The listing builds one solid part. Answer for the finished solid, in the listing's coordinates (mm). A direction names the side the tool comes from. Coordinates: 2 decimals unless noted, no trailing zeros. Write each loop counter-clockwise with the first axis right and the second up, starting at its lowest first coordinate (ties: lowest second). Pieces come first, ordered by that corner, then holes. Notation, with made-up numbers: M 40,23.5 L 69,23.5 A21 ccw 69,27.5 Z; hole C 21,86.5 d10. An arc over 180 degrees is marked long. Answer as CSV lines item,"result". Start each with the question number.
```python
from build123d import *
from build123d.topology import SkipClean

# Parameters (mm, degrees)
CUT_EXTRUDE1_START = -254
CUT_EXTRUDE1_DEPTH = 254
CHAMFER1_SIZE      = 10
CHAMFER2_SIZE      = 10
CHAMFER3_SIZE      = 10
CHAMFER4_SIZE      = 10
FILLET1_R          = 10


with BuildPart() as part:
    # Sketch1 → Revolve4 (revolve)
    with BuildSketch(Plane.XY):
        Polygon((-381, 4.199357945), (-381, 80.399357945), (0, 80.399357945), (0, 105.799357945), (127, 105.799357945), (127, 118.499357945), (431.8, 118.499357945), (431.8, 105.799357945), (482.6, 105.799357945), (482.6, 80.399357945), (685.8, 80.399357945), (685.8, 4.199357945), align=None)
    revolve(axis=Axis((685.8, 4.199357945, 0), (-1, 0, 0)))

    # Sketch3 → Cut-Extrude1 (cut)
    with SkipClean():  # the faces are left unmerged after this step: merging them gives an invalid solid
        with BuildSketch(Plane.ZY.offset(-127).offset(CUT_EXTRUDE1_START)):
            with BuildLine():
                Line((38.1, -89.986362841), (38.1, -103.563715507))
                ThreePointArc((38.1, -103.563715507), (93.3255592, -61.791777823), (114.3, 4.199357945))
                ThreePointArc((114.3, 4.199357945), (93.3255592, 70.190493714), (38.1, 111.962431398))
                Line((38.1, 111.962431398), (38.1, 98.385078732))
                ThreePointArc((38.1, 98.385078732), (84.242269675, 60.995484574), (101.6, 4.199357945))
                ThreePointArc((101.6, 4.199357945), (84.242269675, -52.596768683), (38.1, -89.986362841))
            make_face()
            with BuildLine():
                ThreePointArc((-38.1, 111.962431398), (-114.3, 4.199357945), (-38.1, -103.563715507))
                Line((-38.1, -103.563715507), (-38.1, -89.986362841))
                ThreePointArc((-38.1, -89.986362841), (-101.6, 4.199357945), (-38.1, 98.385078732))
                Line((-38.1, 98.385078732), (-38.1, 111.962431398))
            make_face()
        extrude(amount=CUT_EXTRUDE1_DEPTH, mode=Mode.SUBTRACT)

    # Chamfer1
    chamfer1_edges = [part.edges().sort_by_distance(p)[0] for p in [
        (685.8, -72.000642055, 0),
    ]]
    chamfer(chamfer1_edges, length=CHAMFER1_SIZE)

    # Chamfer2
    chamfer2_edges = [part.edges().sort_by_distance(p)[0] for p in [
        (482.6, -97.400642055, 0),
    ]]
    chamfer(chamfer2_edges, length=CHAMFER2_SIZE)

    # Chamfer3
    chamfer3_edges = [part.edges().sort_by_distance(p)[0] for p in [
        (-381, -72.000642055, 0),
    ]]
    chamfer(chamfer3_edges, length=CHAMFER3_SIZE)

    # Chamfer4
    chamfer4_edges = [part.edges().sort_by_distance(p)[0] for p in [
        (0, -97.400642055, 0),
    ]]
    chamfer(chamfer4_edges, length=CHAMFER4_SIZE)

    # Fillet1
    # the kernel refuses this fillet: 10 mm, written as the material it adds along each edge
    with BuildSketch(Plane(origin=(381, -64.986362841, 38.1), x_dir=(-1, 0, 0), z_dir=(0, -1, 0))) as fillet1_piece_1_section:
        with BuildLine():
            CenterArc((FILLET1_R, -FILLET1_R), FILLET1_R, 90, 90)
            Line((0, -FILLET1_R), (-FILLET1_R * 0.02, -FILLET1_R))
            Line((-FILLET1_R * 0.02, -FILLET1_R), (-FILLET1_R * 0.02, FILLET1_R * 0.02))
            Line((-FILLET1_R * 0.02, FILLET1_R * 0.02), (FILLET1_R, FILLET1_R * 0.02))
            Line((FILLET1_R, FILLET1_R * 0.02), (FILLET1_R, 0))
        make_face()
    fillet1_piece_1 = extrude(amount=63.577352667, mode=Mode.PRIVATE)
    fillet1_piece_1 = fillet1_piece_1 - Plane(origin=(378.747471164, 4.199357945, 0), x_dir=(0, 0.9270248108869475, 0.3750000000000256), z_dir=(1, 0, 0)) * Cylinder(101.6, 168, mode=Mode.PRIVATE)
    fillet1_piece_1 = fillet1_piece_1 & Plane(origin=(378.747471164, 4.199357945, 0), x_dir=(0, 1, 0), z_dir=(1, 0, 0)) * Cylinder(114.3, 168, mode=Mode.PRIVATE)
    add(fillet1_piece_1)
    with BuildSketch(Plane(origin=(381, 136.962431398, 38.1), x_dir=(-1, 0, 0), z_dir=(0, -1, 0))) as fillet1_piece_2_section:
        with BuildLine():
            CenterArc((FILLET1_R, -FILLET1_R), FILLET1_R, 90, 90)
            Line((0, -FILLET1_R), (-FILLET1_R * 0.02, -FILLET1_R))
            Line((-FILLET1_R * 0.02, -FILLET1_R), (-FILLET1_R * 0.02, FILLET1_R * 0.02))
            Line((-FILLET1_R * 0.02, FILLET1_R * 0.02), (FILLET1_R, FILLET1_R * 0.02))
            Line((FILLET1_R, FILLET1_R * 0.02), (FILLET1_R, 0))
        make_face()
    fillet1_piece_2 = extrude(amount=63.577352667, mode=Mode.PRIVATE)
    fillet1_piece_2 = fillet1_piece_2 - Plane(origin=(378.747465839, 4.199357945, 0), x_dir=(0, 0.9270248108869475, 0.3750000000000256), z_dir=(1, 0, 0)) * Cylinder(101.6, 168, mode=Mode.PRIVATE)
    fillet1_piece_2 = fillet1_piece_2 & Plane(origin=(378.747465839, 4.199357945, 0), x_dir=(0, 1, 0), z_dir=(1, 0, 0)) * Cylinder(114.3, 168, mode=Mode.PRIVATE)
    add(fillet1_piece_2)
    with BuildSketch(Plane(origin=(381, 73.385078732, -38.1), x_dir=(-1, 0, 0), z_dir=(0, 1, 0))) as fillet1_piece_3_section:
        with BuildLine():
            CenterArc((FILLET1_R, -FILLET1_R), FILLET1_R, 90, 90)
            Line((0, -FILLET1_R), (-FILLET1_R * 0.02, -FILLET1_R))
            Line((-FILLET1_R * 0.02, -FILLET1_R), (-FILLET1_R * 0.02, FILLET1_R * 0.02))
            Line((-FILLET1_R * 0.02, FILLET1_R * 0.02), (FILLET1_R, FILLET1_R * 0.02))
            Line((FILLET1_R, FILLET1_R * 0.02), (FILLET1_R, 0))
        make_face()
    fillet1_piece_3 = extrude(amount=63.577352667, mode=Mode.PRIVATE)
    fillet1_piece_3 = fillet1_piece_3 - Plane(origin=(378.747465659, 4.199357945, 0), x_dir=(0, -0.9270248108869582, -0.3749999999999992), z_dir=(1, 0, 0)) * Cylinder(101.6, 168, mode=Mode.PRIVATE)
    fillet1_piece_3 = fillet1_piece_3 & Plane(origin=(378.747465659, 4.199357945, 0), x_dir=(0, 1, 0), z_dir=(1, 0, 0)) * Cylinder(114.3, 168, mode=Mode.PRIVATE)
    add(fillet1_piece_3)
    with BuildSketch(Plane(origin=(381, -128.563715507, -38.1), x_dir=(-1, 0, 0), z_dir=(0, 1, 0))) as fillet1_piece_4_section:
        with BuildLine():
            CenterArc((FILLET1_R, -FILLET1_R), FILLET1_R, 90, 90)
            Line((0, -FILLET1_R), (-FILLET1_R * 0.02, -FILLET1_R))
            Line((-FILLET1_R * 0.02, -FILLET1_R), (-FILLET1_R * 0.02, FILLET1_R * 0.02))
            Line((-FILLET1_R * 0.02, FILLET1_R * 0.02), (FILLET1_R, FILLET1_R * 0.02))
            Line((FILLET1_R, FILLET1_R * 0.02), (FILLET1_R, 0))
        make_face()
    fillet1_piece_4 = extrude(amount=63.577352667, mode=Mode.PRIVATE)
    fillet1_piece_4 = fillet1_piece_4 - Plane(origin=(378.747464841, 4.199357945, 0), x_dir=(0, -0.9270248108869582, -0.3749999999999992), z_dir=(1, 0, 0)) * Cylinder(101.6, 168, mode=Mode.PRIVATE)
    fillet1_piece_4 = fillet1_piece_4 & Plane(origin=(378.747464841, 4.199357945, 0), x_dir=(0, 1, 0), z_dir=(1, 0, 0)) * Cylinder(114.3, 168, mode=Mode.PRIVATE)
    add(fillet1_piece_4)
    # the kernel refuses this fillet: 10 mm, written as the material it takes off along each edge
    with BuildSketch(Plane(origin=(127, -64.986362841, 38.1), x_dir=(0, 0, -1), z_dir=(0, -1, 0))) as fillet1_2_piece_1_section:
        with BuildLine():
            CenterArc((FILLET1_R, FILLET1_R), FILLET1_R, 180, 90)
            Line((0, FILLET1_R), (-FILLET1_R * 0.02, FILLET1_R))
            Line((-FILLET1_R * 0.02, FILLET1_R), (-FILLET1_R * 0.02, -FILLET1_R * 0.02))
            Line((-FILLET1_R * 0.02, -FILLET1_R * 0.02), (FILLET1_R, -FILLET1_R * 0.02))
            Line((FILLET1_R, -FILLET1_R * 0.02), (FILLET1_R, 0))
        make_face()
    fillet1_2_piece_1 = extrude(amount=63.577352667, mode=Mode.PRIVATE)
    fillet1_2_piece_1 = fillet1_2_piece_1 - Plane(origin=(129.273265728, 4.199357945, 0), x_dir=(0, 1, 0), z_dir=(1, 0, 0)) * Cylinder(101.6, 168, mode=Mode.PRIVATE)
    fillet1_2_piece_1 = fillet1_2_piece_1 & Plane(origin=(129.273265728, 4.199357945, 0), x_dir=(0, 1, 0), z_dir=(1, 0, 0)) * Cylinder(114.3, 168, mode=Mode.PRIVATE)
    add(fillet1_2_piece_1, mode=Mode.SUBTRACT)
    with BuildSketch(Plane(origin=(127, 136.962431398, 38.1), x_dir=(0, 0, -1), z_dir=(0, -1, 0))) as fillet1_2_piece_2_section:
        with BuildLine():
            CenterArc((FILLET1_R, FILLET1_R), FILLET1_R, 180, 90)
            Line((0, FILLET1_R), (-FILLET1_R * 0.02, FILLET1_R))
            Line((-FILLET1_R * 0.02, FILLET1_R), (-FILLET1_R * 0.02, -FILLET1_R * 0.02))
            Line((-FILLET1_R * 0.02, -FILLET1_R * 0.02), (FILLET1_R, -FILLET1_R * 0.02))
            Line((FILLET1_R, -FILLET1_R * 0.02), (FILLET1_R, 0))
        make_face()
    fillet1_2_piece_2 = extrude(amount=63.577352667, mode=Mode.PRIVATE)
    fillet1_2_piece_2 = fillet1_2_piece_2 - Plane(origin=(129.273255891, 4.199357945, 0), x_dir=(0, 1, 0), z_dir=(1, 0, 0)) * Cylinder(101.6, 168, mode=Mode.PRIVATE)
    fillet1_2_piece_2 = fillet1_2_piece_2 & Plane(origin=(129.273255891, 4.199357945, 0), x_dir=(0, 1, 0), z_dir=(1, 0, 0)) * Cylinder(114.3, 168, mode=Mode.PRIVATE)
    add(fillet1_2_piece_2, mode=Mode.SUBTRACT)
    with BuildSketch(Plane(origin=(127, -128.563715507, -38.1), x_dir=(0, 0, 1), z_dir=(0, 1, 0))) as fillet1_2_piece_3_section:
        with BuildLine():
            CenterArc((FILLET1_R, FILLET1_R), FILLET1_R, 180, 90)
            Line((0, FILLET1_R), (-FILLET1_R * 0.02, FILLET1_R))
            Line((-FILLET1_R * 0.02, FILLET1_R), (-FILLET1_R * 0.02, -FILLET1_R * 0.02))
            Line((-FILLET1_R * 0.02, -FILLET1_R * 0.02), (FILLET1_R, -FILLET1_R * 0.02))
            Line((FILLET1_R, -FILLET1_R * 0.02), (FILLET1_R, 0))
        make_face()
    fillet1_2_piece_3 = extrude(amount=63.577352667, mode=Mode.PRIVATE)
    fillet1_2_piece_3 = fillet1_2_piece_3 - Plane(origin=(129.273255891, 4.199357945, 0), x_dir=(0, 1, 0), z_dir=(1, 0, 0)) * Cylinder(101.6, 168, mode=Mode.PRIVATE)
    fillet1_2_piece_3 = fillet1_2_piece_3 & Plane(origin=(129.273255891, 4.199357945, 0), x_dir=(0, 1, 0), z_dir=(1, 0, 0)) * Cylinder(114.3, 168, mode=Mode.PRIVATE)
    add(fillet1_2_piece_3, mode=Mode.SUBTRACT)
    with BuildSketch(Plane(origin=(127, 73.385078732, -38.1), x_dir=(0, 0, 1), z_dir=(0, 1, 0))) as fillet1_2_piece_4_section:
        with BuildLine():
            CenterArc((FILLET1_R, FILLET1_R), FILLET1_R, 180, 90)
            Line((0, FILLET1_R), (-FILLET1_R * 0.02, FILLET1_R))
            Line((-FILLET1_R * 0.02, FILLET1_R), (-FILLET1_R * 0.02, -FILLET1_R * 0.02))
            Line((-FILLET1_R * 0.02, -FILLET1_R * 0.02), (FILLET1_R, -FILLET1_R * 0.02))
            Line((FILLET1_R, -FILLET1_R * 0.02), (FILLET1_R, 0))
        make_face()
    fillet1_2_piece_4 = extrude(amount=63.577352667, mode=Mode.PRIVATE)
    fillet1_2_piece_4 = fillet1_2_piece_4 - Plane(origin=(129.273265728, 4.199357945, 0), x_dir=(0, 1, 0), z_dir=(1, 0, 0)) * Cylinder(101.6, 168, mode=Mode.PRIVATE)
    fillet1_2_piece_4 = fillet1_2_piece_4 & Plane(origin=(129.273265728, 4.199357945, 0), x_dir=(0, 1, 0), z_dir=(1, 0, 0)) * Cylinder(114.3, 168, mode=Mode.PRIVATE)
    add(fillet1_2_piece_4, mode=Mode.SUBTRACT)


solid = part.part
```
1) For a pull along Z with two mould halves and no side action, classify faces 4 (the face through (452.49, -76.43, 61.82)), 5 (the face through (0, 79.3, -14)) as +Z half, -Z half, draft (parallel to the pull), parting line (faces both ways), or undercut.
2) Find the intervals of material crossed by line 1 (X direction, y = 67, z = 94.5); line 2 (Y direction, x = 182, z = 38); line 3 (Y direction, x = -234, z = 2.5), in increasing order. Write a range as from..to.
3) The part is cut by section D-D (x = 538). Determine the outline of the cut face in (y, z).
4) The part is cut by section A-A (x = 214.5). Determine the outline of the cut face in (y, z), then the cut area to 3 significant figures.
5) The part is cut by section C-C (x = 89.5). Determine the outline of the cut face in (y, z), then the cut area to 3 significant figures.
6) The part is cut by section B-B (z = 0). Determine the outline of the cut face in (x, y), then the cut area to 3 significant figures.
7) Each of these flat-tipped pins is pushed along its axis until it touches: P1, Ø7, axis at x = 207, y = -97, coming from the -Z side; P2, Ø15, axis at x = 268, y = -96.5, coming from the +Z side; P3, Ø1.5, axis at x = 154.5, z = 83, coming from the +Y side. Where does it stop, or does it pass through?
8) Which of the six approach directions +Z, -Z, +X, -X, +Y, -Y give full straight-line access (tool end or side, diameter ignored) to faces 1 (the face through (-182.9, 76.88, -22.89)), 2 (the face through (431.8, -73, 67)), 3 (the face through (381, 5, -103))?
Completed:
1,face 4,"parting line"
1,face 5,"draft"
2,line 1,"381..431.8"
2,line 2,"-103.6..112"
2,line 3,"-71.96..80.36"
3,outline,"C 4.2,0 d152.4"
4,outline,"M -103.56,-38.1 L -89.99,-38.1 A101.6 ccw 98.39,-38.1 L 111.96,-38.1 A114.3 ccw 111.96,38.1 L 98.39,38.1 A101.6 ccw -89.99,38.1 L -103.56,38.1 A114.3 ccw Z"
4,area,"34,400 mm²"
5,outline,"C 4.2,0 d203.2"
5,area,"32,400 mm²"
6,outline,"M -381,-62 L -371,-72 L 0,-72 L 0,-87.4 L 10,-97.4 L 127,-97.4 L 127,-110.1 L 431.8,-110.1 L 431.8,-97.4 L 472.6,-97.4 L 482.6,-87.4 L 482.6,-72 L 675.8,-72 L 685.8,-62 L 685.8,70.4 L 675.8,80.4 L 482.6,80.4 L 482.6,95.8 L 472.6,105.8 L 431.8,105.8 L 431.8,118.5 L 127,118.5 L 127,105.8 L 10,105.8 L 0,95.8 L 0,80.4 L -371,80.4 L -381,70.4 Z"
6,area,"194,000 mm²"
7,P1,"z = -38.1"
7,P2,"z = 40.45"
7,P3,"y = 63.84"
8,face 1,"-X"
8,face 2,"+X"
8,face 3,"-Z, -X"
